Read the model definition and answer for the solid it produces. Units are mm, in the model's axes. Face numbers are marked on the shaded views. Coordinates: 2 decimals unless noted, no trailing zeros. Loops run counter-clockwise (first coordinate to the right, second up) from the corner with the lowest first, then second, coordinate; pieces in that order, holes last. Notation, with made-up numbers: M 45.5,30 L 65.5,30 A8 ccw 65.5,41 Z; hole C 24.25,-22 d1. An arc over 180 degrees is marked long. Put each result on its own line as item: value.
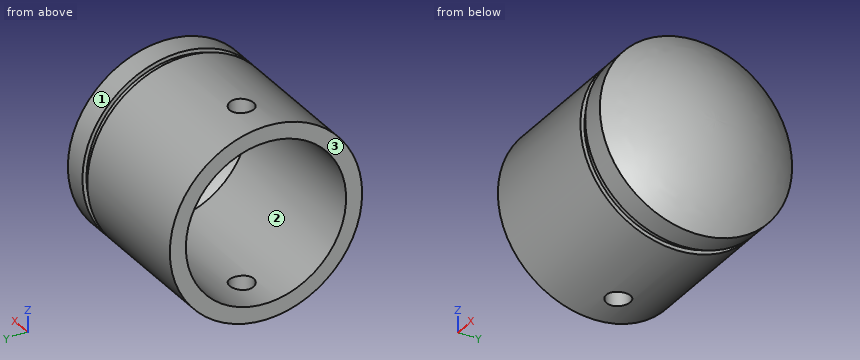
from build123d import *

# Parameters (mm, degrees)
CYLINDER_R     = 3
CYLINDER_DEPTH = 49


with BuildPart() as cylinder:
    # Cylinder → Cylinder (new body)
    with BuildSketch(Plane(origin=(40, 0, -75), x_dir=(1, 0, 0), z_dir=(0, 0, 1))):
        Circle(CYLINDER_R)
    extrude(amount=CYLINDER_DEPTH)


with BuildPart() as piston_hole:
    # Sketch010 → Revolution (revolve)
    with BuildSketch(Plane.XY.offset(-50)):
        with BuildLine():
            Line((30, 20), (70, 20))
            ThreePointArc((76.356083, 0), (74.728852, 10.492854), (70, 20))
            Line((80.356083, 0), (76.356083, 0))
            ThreePointArc((80.356083, 0), (78.207329, 12.706537), (72, 24))
            Line((66, 24), (72, 24))
            Line((66, 23), (66, 24))
            Line((64, 23), (66, 23))
            Line((64, 24), (64, 23))
            Line((30, 24), (64, 24))
            Line((30, 20), (30, 24))
        make_face()
    revolve(axis=Axis((0, 0, -50), (1, 0, 0)))

    # Cut: cut Cylinder
    add(cylinder.part, mode=Mode.SUBTRACT)


solid = piston_hole.part
1) Straight lines are drawn through the part: line 1 (Z direction, x = 34.5, y = 0.5); line 2 (Y direction, x = 63, z = -55); line 3 (X direction, y = 0, z = -28.5). For each, find the intervals that lie inside material, in ascending order. Write a range as [from, to].
Answer list:
line 1: z = [-73.99, -69.99], [-30.01, -26.01]
line 2: y = [-23.47, -19.36], [19.36, 23.47]
line 3: x = [30, 37], [43, 73.82]
2) Find section C-C, the plane y = 1.5. Count the separate pieces of the cut face and the enclosed holes in it, plus the area to 3 significant figures.
Answer list:
separate pieces: 3
enclosed holes: 0
area: 472 mm^2
3) Determine the mould class of the marked faces 1, 2 and 3 for opening direction Y: released by +Y, released by -Y, zero draft, split by the parting line, or undercut.
Answer list:
face 1: split by the parting line
face 2: undercut
face 3: zero draft
4) Find section A-A, the plane x = 46. Write down the section's boundary in (y, z), plus the area to 3 significant figures.
Answer list:
outline: C 0,-50 d48; hole C 0,-50 d40
area: 553 mm^2
5) Given pin 1 Ø14.5 at (y, z) = (-6.5, -56.5) entering from +X; pin 2 Ø8 at (x, y) = (63.5, 0) entering from -Z; pin 3 Ø1.5 at (x, y) = (62, -17) entering from +Z, each flat-ended and moving along its own axis, determine where each tip first touches the part or whether it passes through.
Answer list:
pin 1: stops at x = 80.31
pin 2: stops at z = -74
pin 3: stops at z = -32.34
6) Find section B-B, the plane x = 40. Write down the section's boundary in (y, z), plus the area to 3 significant figures.
Answer list:
outline: M -3,-73.81 L -3,-69.77 A20 cw -3,-30.23 L -3,-26.19 A24 ccw Z; M 3,-73.81 A24 ccw 3,-26.19 L 3,-30.23 A20 cw 3,-69.77 Z
area: 505 mm^2
